CAD build for the part. Positions are in the model's coordinates, mm. A direction names the side the tool comes from. Coordinates: 2 decimals unless noted, no trailing zeros. Order: outer loops, then holes, each group sorted by start corner. A loop starts at its lowest first (then second) coordinate and runs counter-clockwise, first axis right, second up. Notation, with made-up numbers: (48, -19.5) - (97, -19.5) arc R13 cw to (97, -12.5) - close; hole circle Ø9 at (87.5, 57). An arc over 180 degrees is marked (long way). Use one line per item in the form item = value.
```python
from build123d import *

# Parameters (mm, degrees)
BASE_SKETCH_W           = 42
BASE_SKETCH_H           = 20
BASE_DEPTH              = 10
MAGNET_TOWER_SKETCH_W   = 15
MAGNET_TOWER_SKETCH_H   = 11
MAGNET_TOWER_DEPTH      = 20
MAGNET_HOLES_SKETCH_R   = 5.5
MAGNET_HOLES_DEPTH      = 5
MOUNT_SCREW_D           = 6.6
MOUNT_SCREW_CBORE_D     = 11
MOUNT_SCREW_CBORE_DEPTH = 6.4
ROUNDING_R              = 5
PROFILE_CLIP_DEPTH      = 3
PROFILE_CLIP_ANGLE_SIZE = 3


with BuildPart() as part:
    # Base sketch → Base (new body)
    with BuildSketch(Plane.XY):
        Rectangle(BASE_SKETCH_W, BASE_SKETCH_H)
    extrude(amount=BASE_DEPTH)

    # Magnet tower sketch → Magnet tower (add)
    with BuildSketch(Plane.XZ.offset(10)):
        with Locations((-13.5, 15.5)):
            Rectangle(MAGNET_TOWER_SKETCH_W, MAGNET_TOWER_SKETCH_H)
        with Locations((13.5, 15.5)):
            Rectangle(MAGNET_TOWER_SKETCH_W, MAGNET_TOWER_SKETCH_H)
    extrude(amount=-MAGNET_TOWER_DEPTH)

    # Magnet holes sketch → Magnet holes (cut)
    with BuildSketch(Plane.XZ.offset(10)):
        with Locations(Location((-13.5, 14, 0), (0, 0, 270))):
            Circle(MAGNET_HOLES_SKETCH_R)
        with Locations(Location((13.5, 14, 0), (0, 0, 270))):
            Circle(MAGNET_HOLES_SKETCH_R)
    extrude(amount=-MAGNET_HOLES_DEPTH, mode=Mode.SUBTRACT)

    # Mount screw (through all)
    with Locations(Plane.XY.offset(10)):
        with Locations((0, 0)):
            CounterBoreHole(MOUNT_SCREW_D / 2, MOUNT_SCREW_CBORE_D / 2, MOUNT_SCREW_CBORE_DEPTH)

    # Rounding
    rounding_edges = [part.edges().sort_by_distance(p)[0] for p in [
        (-21, 0, 21),
        (-6, 0, 21),
        (21, 0, 21),
        (6, 0, 21),
    ]]
    fillet(rounding_edges, radius=ROUNDING_R)

    # Profile clip sketch → Profile clip (add)
    with BuildSketch(Plane(origin=(0, 0, 0), x_dir=(-1, 0, 0), z_dir=(0, 0, -1))):
        with BuildLine():
            Line((-8.062257748, 4), (-21, 4))
            Line((-21, 4), (-21, -4))
            Line((-21, -4), (-8.062257748, -4))
            ThreePointArc((-8.062257748, -4), (-9, 0), (-8.062257748, 4))
        make_face()
        with BuildLine():
            Line((21, 4), (8.062257748, 4))
            ThreePointArc((8.062257748, 4), (8.762428879, 2.054224947), (9, 0))
            ThreePointArc((9, 0), (8.762428879, -2.054224947), (8.062257748, -4))
            Line((8.062257748, -4), (21, -4))
            Line((21, -4), (21, 4))
        make_face()
    extrude(amount=PROFILE_CLIP_DEPTH)

    # Profile clip angle
    profile_clip_angle_edges = [part.edges().sort_by_distance(p)[0] for p in [
        (-14.531128874, 4, -3),
        (14.531128874, 4, -3),
    ]]
    chamfer(profile_clip_angle_edges, length=PROFILE_CLIP_ANGLE_SIZE - 0.0001)  # a hair under: the kernel refuses the full size


solid = part.part
```
Item 1: 3-axis set-ups, long thin cutter, end or side, ignore diameter. For faces 4 (the face through (6, 0, 13)), 5 (the face through (14, -5, 14)), 6 (the face through (-1.19, -5.37, 6.84)): which of +Z, -Z, +X, -X, +Y, -Y reach the whole face in a straight line?
Derived:
face_4 = +Z, +Y, -Y
face_5 = -Y
face_6 = +Z
Item 2: Drill centre lines: line 1 (X direction, y = -7.8, z = 14); line 2 (X direction, y = 2, z = 12); line 3 (Y direction, x = 0, z = 8.75). Where is each one in solid material? Low to high. Write a range as [from, to].
Derived:
line_1 = [-21, -19], [-8, -6], [6, 8], [19, 21]
line_2 = [-21, -6], [6, 21]
line_3 = [-10, -5.5], [5.5, 10]
Item 3: Drop flat-ended pins along their axis: pin 1 (3.5 mm diameter, centred on x = -15.5, z = 12.5, fed in from -Y); pin 2 (2 mm diameter, centred on x = 0, y = 5.5, fed in from +Z); pin 3 (10.5 mm diameter, centred on x = 0, y = 0, fed in from +Z). Give the stop position or say it passes through.
Derived:
pin_1 = -5
pin_2 = 10
pin_3 = 3.6
Item 4: Cut at B-B, the plane x = 0. Write the cut outline in (y, z).
Derived:
outline = (-10, 0) - (-3.3, 0) - (-3.3, 3.6) - (-5.5, 3.6) - (-5.5, 10) - (-10, 10) - close; (3.3, 0) - (10, 0) - (10, 10) - (5.5, 10) - (5.5, 3.6) - (3.3, 3.6) - close
Item 5: Cut at A-A, the plane z = 14. Write the cut outline in (x, y), plus the area to 3 significant figures.
Derived:
outline = (-21, -10) - (-19, -10) - (-19, -5) - (-8, -5) - (-8, -10) - (-6, -10) - (-6, 10) - (-21, 10) - close; (6, -10) - (8, -10) - (8, -5) - (19, -5) - (19, -10) - (21, -10) - (21, 10) - (6, 10) - close
area = 490 mm²
Item 6: Two-plate mould, pull along X, no slides. Class faces 1 (the face through (-21, 0, 6)), 2 (the face through (2.43, 2.23, 1.77)), 3 (the face through (-14, -4, -1)): +X half, -X half, draft (parallel to the pull), parting line (faces both ways), or undercut.
Derived:
face_1 = -X half
face_2 = undercut
face_3 = draft
Item 7: Cut at C-C, the plane y = -7.5. Write the cut outline in (x, z), plus the area to 3 significant figures.
Derived:
outline = (-21, 0) - (21, 0) - (21, 16) arc R5 ccw to (16, 21) - (11, 21) arc R5 ccw to (6, 16) - (6, 10) - (-6, 10) - (-6, 16) arc R5 ccw to (-11, 21) - (-16, 21) arc R5 ccw to (-21, 16) - close; hole circle Ø11 at (-13.5, 14); hole circle Ø11 at (13.5, 14)
area = 538 mm²
